```python
from build123d import *

# Parameters (mm, degrees)
BOSS_EXTRUDE1_DEPTH      = 30
BOSS_EXTRUDE1_DEPTH_BACK = 30
CUT_EXTRUDE1_DEPTH       = 18
CUT_EXTRUDE1_DEPTH_BACK  = 18
SKETCH3_W                = 21.854352608
SKETCH3_H                = 45
CUT_EXTRUDE2_DEPTH       = 99.234413522
SKETCH4_R                = 1.6
CUT_EXTRUDE3_DEPTH       = 84.366660003
SKETCH6_W                = 48
SKETCH6_H                = 4
CUT_EXTRUDE5_DEPTH       = 2
SKETCH9_W                = 22
SKETCH9_H                = 60
CUT_EXTRUDE7_DEPTH       = 84.366660003
SKETCH10_W               = 66
SKETCH10_H               = 25
SKETCH10_H_2             = 60
SKETCH10_W_2             = 19
SKETCH10_H_3             = 36
BOSS_EXTRUDE2_DEPTH      = 5
SKETCH11_R               = 1.6
CUT_EXTRUDE8_DEPTH       = 88.82938005
SKETCH13_W               = 24.8
SKETCH13_H               = 30
BOSS_EXTRUDE3_DEPTH      = 27.15
SKETCH14_W               = 16.4
SKETCH14_H               = 16.4
SKETCH14_W_2             = 16
SKETCH14_H_2             = 16
CUT_EXTRUDE9_DEPTH       = 12
SKETCH15_W               = 56
SKETCH15_H               = 50
CUT_EXTRUDE10_DEPTH      = 45


with BuildPart() as part:
    # Sketch1 → Boss-Extrude1 (new, two sides)
    with BuildSketch(Plane.XY) as boss_extrude1_sk:
        with BuildLine():
            Line((55, 0), (-55, 0))
            ThreePointArc((-55, 0), (0, -55), (55, 0))
        make_face()
    extrude(amount=BOSS_EXTRUDE1_DEPTH)
    extrude(boss_extrude1_sk.sketch, amount=-BOSS_EXTRUDE1_DEPTH_BACK)

    # Sketch2 → Cut-Extrude1 (cut, two sides)
    with BuildSketch(Plane.XY) as cut_extrude1_sk:
        Polygon((0, 0), (-9.5, 0), (-9.5, -52), (2.8860755, -52), (9.5, -52), (9.5, 0), align=None)
    extrude(amount=CUT_EXTRUDE1_DEPTH, mode=Mode.SUBTRACT)
    extrude(cut_extrude1_sk.sketch, amount=-CUT_EXTRUDE1_DEPTH_BACK, mode=Mode.SUBTRACT)

    # Sketch3 → Cut-Extrude2 (cut, through all)
    with BuildSketch(Plane.XY.offset(30)):
        with Locations((-43.927176304, -26.5)):
            Rectangle(SKETCH3_W, SKETCH3_H)
        with Locations((43.927176304, -26.5)):
            Rectangle(SKETCH3_W, SKETCH3_H)
    extrude(amount=-CUT_EXTRUDE2_DEPTH, mode=Mode.SUBTRACT)

    # Sketch4 → Cut-Extrude3 (cut, through all)
    with BuildSketch(Plane(origin=(0, 0, 0), x_dir=(1, 0, 0), z_dir=(0, 1, 0))):
        with Locations(Location((45, 20, 0), (0, 0, 270))):
            Circle(SKETCH4_R)
        with Locations(Location((45, -20, 0), (0, 0, 180))):
            Circle(SKETCH4_R)
        with Locations(Location((-45, -20, 0), (0, 0, 270))):
            Circle(SKETCH4_R)
        with Locations(Location((-45, 20, 0), (0, 0, 270))):
            Circle(SKETCH4_R)
    extrude(amount=-CUT_EXTRUDE3_DEPTH, mode=Mode.SUBTRACT)

    # Sketch6 → Cut-Extrude5 (cut)
    with BuildSketch(Plane(origin=(33, 0, 0), x_dir=(0, 0, -1), z_dir=(1, 0, 0))):
        with Locations((0, -18)):
            Rectangle(SKETCH6_W, SKETCH6_H)
    extrude(amount=-CUT_EXTRUDE5_DEPTH, mode=Mode.SUBTRACT)

    # Sketch9 → Cut-Extrude7 (cut, through all)
    with BuildSketch(Plane(origin=(0, 0, 0), x_dir=(1, 0, 0), z_dir=(0, 1, 0))):
        with Locations((-44, 0)):
            Rectangle(SKETCH9_W, SKETCH9_H)
        with Locations((44, 0)):
            Rectangle(SKETCH9_W, SKETCH9_H)
    extrude(amount=-CUT_EXTRUDE7_DEPTH, mode=Mode.SUBTRACT)

    # Sketch10 → Boss-Extrude2 (add)
    with BuildSketch(Plane(origin=(0, 0, 0), x_dir=(1, 0, 0), z_dir=(0, 1, 0))):
        with Locations((0, 42.5)):
            Rectangle(SKETCH10_W, SKETCH10_H)
        Rectangle(SKETCH10_W, SKETCH10_H_2)
        Rectangle(SKETCH10_W_2, SKETCH10_H_3, mode=Mode.SUBTRACT)
        with Locations((0, -42.5)):
            Rectangle(SKETCH10_W, SKETCH10_H)
    extrude(amount=BOSS_EXTRUDE2_DEPTH)

    # Sketch11 → Cut-Extrude8 (cut, through all)
    with BuildSketch(Plane(origin=(0, 5, 0), x_dir=(1, 0, 0), z_dir=(0, 1, 0))):
        with Locations(Location((-20, 35, 0), (0, 0, 270))):
            Circle(SKETCH11_R)
        with Locations(Location((20, 35, 0), (0, 0, 270))):
            Circle(SKETCH11_R)
        with Locations(Location((-20, -35, 0), (0, 0, 270))):
            Circle(SKETCH11_R)
        with Locations(Location((20, -35, 0), (0, 0, 270))):
            Circle(SKETCH11_R)
    extrude(amount=-CUT_EXTRUDE8_DEPTH, mode=Mode.SUBTRACT)

    # Sketch13 → Boss-Extrude3 (add)
    with BuildSketch(Plane(origin=(0, 0, -30), x_dir=(-1, 0, 0), z_dir=(0, 0, -1))):
        with Locations((0, -15)):
            Rectangle(SKETCH13_W, SKETCH13_H)
    boss_extrude3 = extrude(amount=BOSS_EXTRUDE3_DEPTH)

    # Sketch14 → Cut-Extrude9 (cut)
    with BuildSketch(Plane(origin=(0, 0, -57.15), x_dir=(-1, 0, 0), z_dir=(0, 0, -1))):
        with Locations((0, -17)):
            Rectangle(SKETCH14_W, SKETCH14_H)
        with Locations((0, -17)):
            Rectangle(SKETCH14_W_2, SKETCH14_H_2, mode=Mode.SUBTRACT)
        with Locations((0, -17)):
            Rectangle(SKETCH14_W_2, SKETCH14_H_2)
    cut_extrude9 = extrude(amount=-CUT_EXTRUDE9_DEPTH, mode=Mode.SUBTRACT)

    # Mirror2: Boss-Extrude3 across plane
    add(boss_extrude3.mirror(Plane(origin=(0, 0, 0), x_dir=(1, 0, 0), z_dir=(0, 0, -1))))

    # Mirror3: Cut-Extrude9 across plane
    add(cut_extrude9.mirror(Plane(origin=(0, 0, 0), x_dir=(1, 0, 0), z_dir=(0, 0, -1))), mode=Mode.SUBTRACT)

    # Sketch15 → Cut-Extrude10 (cut)
    with BuildSketch(Plane(origin=(0, 5, 0), x_dir=(1, 0, 0), z_dir=(0, 1, 0))):
        Rectangle(SKETCH15_W, SKETCH15_H)
    extrude(amount=-CUT_EXTRUDE10_DEPTH, mode=Mode.SUBTRACT)


solid = part.part
```
Design review of the part built by this model. Coordinates are the model's own, in mm. A direction names the side the tool comes from. Coordinates: 2 decimals unless noted, no trailing zeros. Order: outer loops, then holes, each group sorted by start corner. A loop starts at its lowest first (then second) coordinate and runs counter-clockwise, first axis right, second up.
1) Take a section at C-C, the plane x = -20. Give the boundary of the cut face in (y, z), and give its area (3 significant figures).
2) Mouldability with a two-part tool opening along Z and no side actions: class faces 5 (the flat face through (0, -17, -45.15)), 6 (the flat face through (23, 0, -43)), 7 (the flat face through (0, -17, 25)) as +Z half, -Z half, draft (parallel to the pull), parting line (faces both ways), or undercut.
3) For faces 1 (the flat face through (0, -52, 0)), 2 (the flat face through (0, 2, -55)), 3 (the flat face through (-8.2, -17, -51)), 4 (the flat face through (0, -17, 45.15)), list the 3-axis set-ups (+Z, -Z, +X, -X, +Y, -Y) from which the entire face can be reached by the end or side of a thin tool; tool diameter is ignored.
4) Clearance check with flat-ended pins moving along their axes: pin 1 (3.5 mm diameter, centred on x = 2.5, y = -43, fed in from -Z); pin 2 (15 mm diameter, centred on x = -10, z = -4.5, fed in from +Y); pin 3 (1.5 mm diameter, centred on x = 3.5, y = -22, fed in from -Z). State where each tip first meets the part, or that it passes through.
5) Take a section at D-D, the plane z = 4.5. Give the boundary of the cut face in (x, y).
6) Wall thickness on line 1 along X through (y, z) = (3.8, -35); line 2 along X through (y, z) = (-22, 15.5); line 3 along Z through (x, y) = (24, -25): over which ranges is each line inside the solid? List them lowest first.
7) Take a section at A-A, the plane z = -35. Give the boundary of the cut face in (x, y).
8) Take a section at B-B, the plane y = -5. Give the boundary of the cut face in (x, z).
Returned:
1. outline: (-51.23, -30) - (0, -30) - (0, -33.4) - (5, -33.4) - (5, -25) - (-40, -25) - (-40, 25) - (5, 25) - (5, 33.4) - (0, 33.4) - (0, 30) - (-51.23, 30) - close; (0, -55) - (5, -55) - (5, -36.6) - (0, -36.6) - close; (0, 36.6) - (5, 36.6) - (5, 55) - (0, 55) - close
1. area: 1,340 mm2
2. face 5: -Z half
2. face 6: draft
2. face 7: undercut
3. face 1: +Y
3. face 2: -Z, +X, -X, +Y
3. face 3: -Z
3. face 4: +Z
4. pin 1: stops at z = -30
4. pin 2: stops at y = -40
4. pin 3: stops at z = -45.15
5. outline: (-33, -44) arc R55 ccw to (33, -44) - (33, -20) - (31, -20) - (31, -16) - (33, -16) - (33, 5) - (28, 5) - (28, -40) - (9.5, -40) - (9.5, -52) - (-9.5, -52) - (-9.5, -40) - (-28, -40) - (-28, 5) - (-33, 5) - close
6. line 1: x = -33 to -21.6, -18.4 to 18.4, 21.6 to 33
6. line 2: x = -33 to -28, 28 to 33
6. line 3: z = -30 to -25, 25 to 30
7. outline: (-33, 0) - (-21.6, 0) - (-21.6, 5) - (-33, 5) - close; (-18.4, 0) - (-12.4, 0) - (-12.4, -30) - (12.4, -30) - (12.4, 0) - (18.4, 0) - (18.4, 5) - (-18.4, 5) - close; (21.6, 0) - (33, 0) - (33, 5) - (21.6, 5) - close
8. outline: (-33, -30) - (-12.4, -30) - (-12.4, -57.15) - (12.4, -57.15) - (12.4, -30) - (33, -30) - (33, 30) - (12.4, 30) - (12.4, 57.15) - (-12.4, 57.15) - (-12.4, 30) - (-33, 30) - close; hole (-28, -25) - (28, -25) - (28, 25) - (-28, 25) - close
